Verification items for the finished model (mm, model axes). Give positions to 0.01 mm unless a question says otherwise; leave off trailing zeros. Order: outer loops, then holes, each group sorted by start corner. A loop starts at its lowest first (then second) coordinate and runs counter-clockwise, first axis right, second up. Notation, with made-up numbers: (53, -8) -> (71, -8) arc R14 cw to (71, 1) -> close; hole circle Ø7 at (54, -13.5). An arc over 180 degrees is marked (long way). One line per question, with ' | ' between items. Start each with the question number.
Q1. Material ranges on probe 1 along Z at (x, y) = (107, -84.3); probe 2 along Z at (x, y) = (99, -83.9); probe 3 along Z at (x, y) = (24.5, -85), recorded low to high. Write a range as [from, to].
Q2. Section check A-A on z = 36. Record the cut outline in (x, y), plus the area to 3 significant figures.
Q3. Section check B-B on y = -84.65. Give the number of separate pieces and of enclosed holes in the cut face, plus the area to 3 significant figures.
Q4. Go/stop test with a flat-tipped pin: pin 1 (6 mm diameter, centred on x = 69, z = 30, fed in from +Y). Record where the tip stops, or that it passes through.
from build123d import *

# Parameters (mm, degrees)
SKETCH009_R             = 1.6
PAD006_DEPTH            = 3
SKETCH010_W             = 25
SKETCH010_H             = 70
POCKET003_DEPTH         = 3.001
SKETCH011_R             = 1.85
POCKET004_DEPTH         = 3.001
SKETCH012_R             = 1.6
SKETCH012_W             = 3.2
SKETCH012_H             = 5.2
POCKET005_DEPTH         = 3.001
SKETCH013_R             = 1.85
POCKET006_DEPTH         = 3.001
SKETCH017_R             = 7
SKETCH017_R_2           = 5
SKETCH017_W             = 15
SKETCH017_H             = 25
POCKET010_DEPTH         = 3.001
BODY003_PLACEMENT_ANGLE = 90


with BuildPart() as part:
    # Sketch009 → Pad006 (new body)
    with BuildSketch(Plane.XZ):
        with BuildLine():
            Line((-59.69, 103.52), (59.69, 103.52))
            ThreePointArc((69.69, 93.52), (66.761068, 100.591068), (59.69, 103.52))
            Line((69.69, 93.52), (69.69, -93.52))
            ThreePointArc((59.69, -103.52), (66.761068, -100.591068), (69.69, -93.52))
            Line((59.69, -103.52), (-59.69, -103.52))
            ThreePointArc((-69.69, -93.52), (-66.761068, -100.591068), (-59.69, -103.52))
            Line((-69.69, -93.52), (-69.69, 93.52))
            ThreePointArc((-59.69, 103.52), (-66.761068, 100.591068), (-69.69, 93.52))
        make_face()
        with Locations((-59.69, 93.52)):
            Circle(SKETCH009_R, mode=Mode.SUBTRACT)
        with Locations((59.69, 93.52)):
            Circle(SKETCH009_R, mode=Mode.SUBTRACT)
        with Locations((59.69, -93.52)):
            Circle(SKETCH009_R, mode=Mode.SUBTRACT)
        with Locations((-59.69, -93.52)):
            Circle(SKETCH009_R, mode=Mode.SUBTRACT)
    extrude(amount=PAD006_DEPTH)

    # Sketch010 → Pocket003 (cut, through all)
    with BuildSketch(Plane.XZ):
        with Locations((-57.19, 0)):
            Rectangle(SKETCH010_W, SKETCH010_H)
        with Locations((57.19, 0)):
            Rectangle(SKETCH010_W, SKETCH010_H)
    extrude(amount=POCKET003_DEPTH, mode=Mode.SUBTRACT)

    # Sketch011 → Pocket004 (cut, through all)
    with BuildSketch(Plane.XZ):
        with Locations((9, 85)):
            Circle(SKETCH011_R)
        with Locations((64, 85)):
            Circle(SKETCH011_R)
        with Locations((64, 50)):
            Circle(SKETCH011_R)
        with Locations((9, 50)):
            Circle(SKETCH011_R)
    extrude(amount=POCKET004_DEPTH, mode=Mode.SUBTRACT)

    # Sketch012 (on Face4 of Pocket004) → Pocket005 (cut, through all)
    with BuildSketch(Plane.XZ.offset(3)):
        with Locations((-53.4, -69)):
            Circle(SKETCH012_R)
        with Locations((3.6, -69)):
            Circle(SKETCH012_R)
        with Locations((46.8, -69)):
            Circle(SKETCH012_R)
        with Locations((-53.4, -45.4)):
            Rectangle(SKETCH012_W, SKETCH012_H)
        with Locations((3.6, -45.4)):
            Rectangle(SKETCH012_W, SKETCH012_H)
        with Locations((3.6, -92.6)):
            Rectangle(SKETCH012_W, SKETCH012_H)
        with Locations((-53.4, -92.6)):
            Rectangle(SKETCH012_W, SKETCH012_H)
        with Locations((46.8, -45.4)):
            Rectangle(SKETCH012_W, SKETCH012_H)
        with Locations((46.8, -92.6)):
            Rectangle(SKETCH012_W, SKETCH012_H)
    extrude(amount=-POCKET005_DEPTH, mode=Mode.SUBTRACT)

    # Sketch013 (on Face4 of Pocket005) → Pocket006 (cut, through all)
    with BuildSketch(Plane.XZ.offset(3)):
        with Locations((-25, 30)):
            Circle(SKETCH013_R)
        with Locations((0, 30)):
            Circle(SKETCH013_R)
        Circle(SKETCH013_R)
        with Locations((-25, 0)):
            Circle(SKETCH013_R)
    extrude(amount=-POCKET006_DEPTH, mode=Mode.SUBTRACT)

    # Sketch017 → Pocket010 (cut, through all)
    with BuildSketch(Plane(origin=(0, 0, 0), x_dir=(1, 0, 0), z_dir=(0, 1, 0))):
        with Locations((9, -38)):
            Circle(SKETCH017_R)
        with Locations((-31, -38)):
            Circle(SKETCH017_R_2)
        with Locations((1.5, -67.5)):
            Rectangle(SKETCH017_W, SKETCH017_H)
    extrude(amount=-POCKET010_DEPTH, mode=Mode.SUBTRACT)


with BuildPart() as part_1:
    # Body003 placement: moved
    add(part.part.moved(Location((69, -83, 5))).rotate(Axis((69, -83, 5), (0, 1, 0)), BODY003_PLACEMENT_ANGLE))


solid = part_1.part
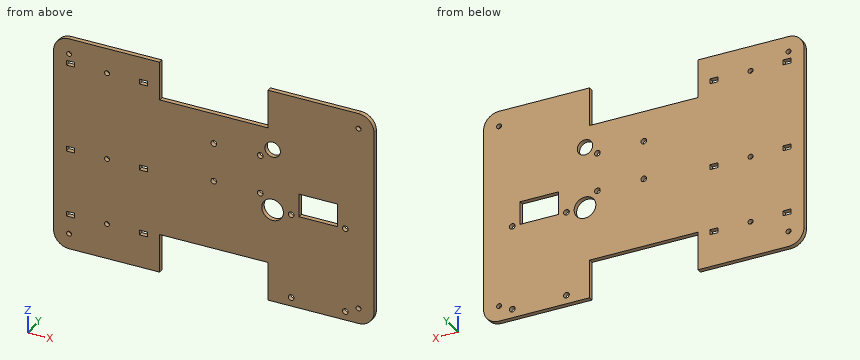
Filled in:
1) probe 1: [-64.69, -11], [3, 31], [41, 74.69] | probe 2: [-39.69, 3.15], [6.85, 28.15], [31.85, 49.69] | probe 3: [-64.69, -43.4], [-40.2, -0.2], [3, 56.8], [60, 74.69]
2) outline: (-34.52, -86) -> (102, -86) -> (102, -83) -> (-34.52, -83) -> close; (112, -86) -> (172.52, -86) -> (172.52, -83) -> (112, -83) -> close | area: 591 mm²
3) separate pieces: 1 | enclosed holes: 24 | area: 24,400 mm²
4) pin 1: y = -83
